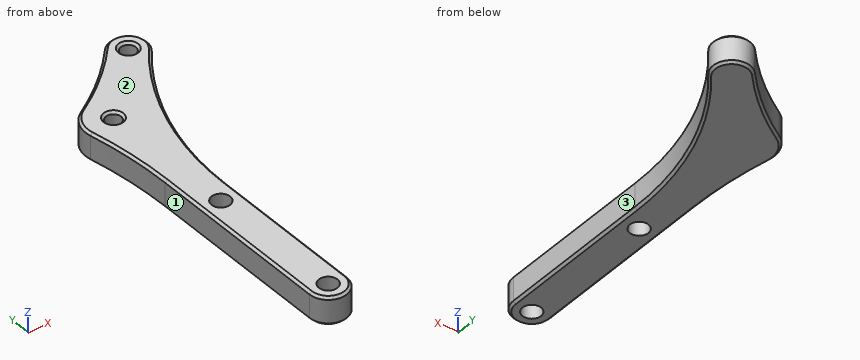
Solid Edge part; units mm, degrees
sketch "Sketch1" plane through (0, 0, 0) normal (0, 0, 1) x (1, 0, 0)
  arc A0 (17.2583, 11.6342) -> (4, -25.9851) centre (64, -25.9851) ccw
  line L0 (4, -60) -> (4, -25.9851)
  line L1 (-4, -60) -> (-4, -19.5959)
  arc A1 (-4, -19.5959) -> (-5.8763, -1.2121) centre (-95, -19.5959) ccw
  arc A2 (11.1633, 16.8117) -> (-3.0473, 5.1686) centre (-33.5198, 56.8544) cw
  arc A3 (4, -60) -> (-4, -60) centre (0, -60) cw
  arc A4 (-5.8763, -1.2121) -> (-3.0473, 5.1686) centre (0, 0) cw
  arc A5 (11.1633, 16.8117) -> (17.2583, 11.6342) centre (14.1421, 14.1421) cw
extrude "Protrusion1" add sketch "Sketch1" along normal blind 6
sketch "Sketch2" plane through (7.8388, -21.1612, 6) normal (0, 0, 1) x (0, 1, 0)
  circle A0 centre (21.1612, 7.8388) radius 1.625
  circle A1 centre (35.3033, -6.3033) radius 1.625
extrude "VaciadoExtruido_1" cut sketch "Sketch2" against normal blind 5
sketch "Sketch3" plane through (7.8388, -21.1612, 6) normal (0, 0, 1) x (0, 1, 0)
  circle A0 centre (-38.8388, 7.8388) radius 2
  circle A1 centre (-8.8388, 7.8388) radius 2
extrude "Cutout1" cut sketch "Sketch3" against normal through all
chamfer "Chaflán_1" distance 0.5 angle 45 18 edges at (4, -42.9925, 6) (0, -64, 6) (-4, -39.798, 6) (-4.4703, -10.3563, 6) (-5.485, 2.4319, 6) (4.5063, 10.443, 6) (16.7318, 17.1907, 6) (7.4116, -6.0415, 6) (4, -42.9925, 0) (0, -64, 0) (-4, -39.798, 0) (-4.4703, -10.3563, 0) (-5.485, 2.4319, 0) (4.5063, 10.443, 0) (16.7318, 17.1907, 0) (7.4116, -6.0415, 0) (0, -1.625, 6) (14.1421, 12.5171, 6)
Build history of the part. All positions in model axes, mm. Face numbers are marked on the shaded views. A direction names the side the tool comes from. Give positions to 0.01 mm unless a question says otherwise; leave off trailing zeros. Loops run counter-clockwise (first coordinate to the right, second up) from the corner with the lowest first, then second, coordinate; pieces in that order, holes last.
1) Band-saw the part on D-D on x = 0. State how many separate pieces and enclosed holes the cut face has, then the cut area to 3 significant figures.
Values follow:
separate pieces: 3
enclosed holes: 0
area: 361 mm2
2) Band-saw the part on B-B on z = 2. List the corners of the cut face in (x, y) (3 decimals), then the cut area to 3 significant figures.
Values follow:
outline: (-5.876, -1.212) arc R91 cw to (-4, -19.596) - (-4, -60) arc R4 ccw to (4, -60) - (4, -25.985) arc R60 cw to (17.258, 11.634) arc R4 ccw to (11.163, 16.812) arc R60 cw to (-3.047, 5.169) arc R6 ccw to start; hole circle Ø4 at (0, -60); hole circle Ø4 at (0, -30); hole circle Ø3.25 at (0, 0); hole circle Ø3.25 at (14.142, 14.142)
area: 750 mm2
3) Probe line 1 along Y through (x, z) = (0, 3.15) (3 decimals); line 2 along Y through (x, z) = (-1, 2.75); line 3 along X through (y, z) = (-30, 2.1). List the from-to ranges inside material, lowest first.
Values follow:
line 1: y = -64 to -62, -58 to -32, -28 to -1.625, 1.625 to 7.091
line 2: y = -63.87 to -61.73, -58.27 to -31.73, -28.27 to -1.28, 1.28 to 6.43
line 3: x = -4 to -2, 2 to 4
4) Band-saw the part on C-C on y = -40. List the corners of the cut face in (x, z), then the cut area to 3 significant figures.
Values follow:
outline: (-4, 0.5) - (-3.5, 0) - (3.5, 0) - (4, 0.5) - (4, 5.5) - (3.5, 6) - (-3.5, 6) - (-4, 5.5) - close
area: 47.5 mm2
5) Band-saw the part on A-A on y = -30. List the corners of the cut face in (x, z).
Values follow:
outline: (-4, 0.5) - (-3.5, 0) - (-2, 0) - (-2, 6) - (-3.5, 6) - (-4, 5.5) - close; (2, 0) - (3.5, 0) - (4, 0.5) - (4, 5.5) - (3.5, 6) - (2, 6) - close
6) 3-axis set-ups, long thin cutter, end or side, ignore diameter. For the marked faces 1, 2 and 3: which of +Z, -Z, +X, -X, +Y, -Y reach the whole face in a straight line?
Values follow:
face 1: +Z, -Z, -X, -Y
face 2: +Z, +X, -X, +Y, -Y
face 3: +Z, -Z, +X, -Y
7) Drop flat-ended pins along their axis: P1, Ø3.5, axis at x = 14.14, y = 14.14, coming from the +Z side; P2, Ø5, axis at x = 9, y = 4, coming from the -Z side; P3, Ø2.5, axis at y = -30, z = 4, coming from the -X side; P4, Ø1.5, axis at y = -18, z = 2.5, coming from the +X side. Give the stop position or say it passes through.
Values follow:
P1: stops at z = 5.63
P2: stops at z = 0
P3: stops at x = -4
P4: stops at x = 4.64
